Geometry check sheet. Reference: the model listing, model coordinates, mm. Give positions to 0.01 mm unless a question says otherwise; leave off trailing zeros. Loops run counter-clockwise (first coordinate to the right, second up) from the corner with the lowest first, then second, coordinate; pieces in that order, holes last. Notation, with made-up numbers: (5.25, -23) -> (58.25, -23) arc R28 ccw to (58.25, 10) -> close; hole circle Ø10 at (56, 37). An arc over 180 degrees is marked (long way). Answer as a JSON object with one key per item and string values.
from build123d import *

# Parameters (mm, degrees)
F0_R     = 76.2
F1_DEPTH = 19.05
F2_R     = 15.6543846093
F3_DEPTH = 19.051
F4_R     = 6.35


with BuildPart() as f1:
    # F0 (on Top) → F1 (new body)
    with BuildSketch(Plane.XY):
        with Locations((-0.2828244178, 0.0797724133)):
            Circle(F0_R)
    extrude(amount=F1_DEPTH)

    # F2 (on face) → F3 (cut, through all)
    with BuildSketch(Plane.XY.offset(19.05)):
        with Locations((0.221362061, 0.4437770694)):
            Circle(F2_R)
    extrude(amount=-F3_DEPTH, mode=Mode.SUBTRACT)

    # F4
    f4_edges = [f1.edges().sort_by_distance(p)[0] for p in [
        (-76.482824, 0.079772, 19.05),
        (-15.433023, 0.443777, 19.05),
    ]]
    fillet(f4_edges, radius=F4_R)


solid = f1.part
1) Draft check along Y on faces 1 (the face through (-17, -14, 19.05)), 2 (the face through (-12.201, -9.082, 6.439)), 3 (the face through (72.398, 22.968, 6.261)). Enter one of: pulls with the +Y half, pulls with the -Y half, needs draft (parallel to the pull), parting line crosses it, or undercut.
Geometry check:
{"face 1": "needs draft", "face 2": "undercut", "face 3": "parting line crosses it"}
2) Section check A-A on z = 14.5. Record the cut outline in (x, y).
Geometry check:
{"outline": "circle Ø151.88 at (-0.28, 0.08); hole circle Ø31.83 at (0.22, 0.44)"}
3) Depth check by flat-ended pin: P1, Ø1.5, axis at y = 26, z = 9, coming from the -X side; P2, Ø10, axis at y = 52.5, z = 5.5, coming from the -X side; P3, Ø25, axis at x = 0.22, y = 0.44, coming from the +Z side; P4, Ø4, axis at y = -7.5, z = 7, coming from the -X side. Enter the tip coordinate at first touch or a pass-through.
Geometry check:
{"P1": "stops at x = -72.21", "P2": "stops at x = -59.93", "P3": "passes through", "P4": "stops at x = -76.28"}
4) Material ranges on line 1 along Y through (x, z) = (-11.5, 8.5); line 2 along Y through (x, z) = (7, 6.75); line 3 along X through (y, z) = (13.5, 4.5), recorded low to high. Write a range as from..to.
Geometry check:
{"line 1": "y = -75.29..-9.93, 10.82..75.45", "line 2": "y = -75.77..-13.67, 14.55..75.93", "line 3": "x = -75.29..-8.42, 8.86..74.73"}
